Geometry check sheet. Reference: the model listing, model coordinates, mm. A direction names the side the tool comes from. Give positions to 0.01 mm unless a question says otherwise; leave off trailing zeros. Order: outer loops, then holes, each group sorted by start corner. A loop starts at its lowest first (then second) coordinate and runs counter-clockwise, first axis right, second up. Notation, with made-up numbers: M -10,63.25 L 35,63.25 A19 cw 35,86.25 Z; hole C 58.5,87 d5. An arc over 180 degrees is marked long. Answer as CSV lines item,"result". Start each with the question number.
Q1. Section check D-D, the plane x = 40. Record the boundary of the cut face in (y, z), then the cut area to 3 significant figures.
Q2. Mould release check, pull along Y, two halves, no side actions. Record for faces 4 (the cylindrical face through (4.4, 44.5, 1.2)), 5 (the flat face through (63, 2, 10)), 6 (the flat face through (20, 6.5, 10)): +Y half, -Y half, draft (parallel to the pull), parting line (faces both ways), or undercut.
Q3. Section check C-C, the plane z = 5.5. Record the boundary of the cut face in (x, y).
Q4. Section check B-B, the plane x = 4.5. Record the boundary of the cut face in (y, z).
Q5. Thickness scan on line 1 (Y direction, x = 4.5, z = 1.85); line 2 (X direction, y = 40, z = 19.25); line 3 (X direction, y = 7, z = 6.5). Record the ranges inside material, lowest first.
Q6. Set-up check for faces 1 (the flat face through (26, 25, 8)), 2 (the flat face through (18, 9, 10)), 3 (the flat face through (21, 9, 10)): record each of +Z, -Z, +X, -X, +Y, -Y from which the full face is reachable in a straight line by a thin tool's end or side.
Q7. Go/stop test with flat-tipped pins: pin 1 (4.5 mm diameter, centred on x = 19, z = 10.5, fed in from +Y); pin 2 (6.5 mm diameter, centred on x = 16.5, y = 9, fed in from +Z); pin 3 (3 mm diameter, centred on x = 61.5, z = 11, fed in from +Y); pin 4 (1 mm diameter, centred on x = 23, y = 25.5, fed in from +Z). Record where each tip stops, or that it passes through.
Q8. Section check A-A, the plane y = 22. Record the boundary of the cut face in (x, z).
Autodesk Inventor part; units mm, degrees
ref_plane "YZ Plane" through (0, 0, 0) normal (1, 0, 0) x (0, 1, 0)
ref_plane "XZ Plane" through (0, 0, 0) normal (0, 1, 0) x (-1, 0, 0)
ref_plane "XY Plane" through (0, 0, 0) normal (0, 0, 1) x (1, 0, 0)
sketch "Sketch1" plane through (0, 0, 0) normal (0, 0, 1) x (1, 0, 0)
  line L0 (0, 0) -> (0, 40)
  line L1 (0, 0) -> (63, 0)
  line L2 (63, 0) -> (63, 5)
  line L3 (63, 5) -> (9, 5)
  arc A0 (9, 40) -> (0, 40) centre (4.5, 40) ccw
  line L4 (9, 40) -> (9, 5)
  circle A1 centre (4.5, 40) radius 2.5
  dimension "d0" = 40
  dimension "d2" = 5
  dimension "d6" = 4.5
  dimension "d7" = 5
  dimension "d8" = 9
  dimension "d9" = 54
  dimension "d47" = 32.5
extrude "Extrusion1" add sketch "Sketch1" along normal blind 20
sketch "Sketch2" plane through (9, 5, 0) normal (0, 1, 0) x (1, 0, 0)
  line L0 (0, 0) -> (0, -20)
  circle A0 centre (26, -10) radius 10
  line L1 (0, 0) -> (54, 0)
  circle A1 centre (52, -10) radius 2
  line L2 (54, 0) -> (54, -20)
  point P0 (-9, 0)
  dimension "d14" = 20
  dimension "d16" = 26
  dimension "d20" = 4
  dimension "d21" = 10
  dimension "d22" = 14
sketch "Sketch6" plane through (9, 5, 0) normal (1, 0, 0) x (0, 0, -1)
  point P0 (0, -5)
sketch "Sketch7" plane through (9, 5, 0) normal (1, 0, 0) x (0, 0, -1)
  line L0 (-10, 41.0364) -> (-10, 39.6436)
  line L1 (0, 39.5) -> (-20, 39.5)
  line L2 (-2.5, 39.5) -> (-2.5, 25.5)
  line L3 (-17.5, 39.5) -> (-17.5, 25.5)
  line L4 (-17.5, 39.5) -> (-2.5, 39.5)
  line L5 (0, 32.5) -> (-20, 32.5)
  line L6 (-17.5, 25.5) -> (-2.5, 25.5)
  point P0 (0, -5)
  dimension "d40" = 14
  dimension "d41" = 14
  dimension "d42" = 15
extrude "Extrusion5" cut sketch "Sketch7" against normal blind 14
sketch "Sketch8" plane through (0, 0, 0) normal (0, 0, -1) x (-1, 0, 0)
  point P0 (0, 0)
extrude "Extrusion6" add sketch "Sketch2" along normal blind 20
sketch "Sketch9" plane through (35, 25, 10) normal (0, 1, 0) x (1, 0, 0)
  circle A0 centre (0, 0) radius 9
  point P0 (-35, 10)
  dimension "d50" = 18
extrude "Extrusion7" cut sketch "Sketch9" against normal blind 25
sketch "Sketch10" plane through (9, 5, 20) normal (0, 1, 0) x (1, 0, 0)
  line L0 (6, 8) -> (12, 8)
  line L1 (12, 8) -> (12, 12)
  line L2 (12, 12) -> (6, 12)
  line L3 (6, 12) -> (6, 8)
  line L4 (26, 0) -> (0, 0)
  line L5 (0, 2.5) -> (0, 17.5)
  point P0 (-9, 20)
  dimension "d53" = 6
  dimension "d54" = 4
  dimension "d55" = 8
  dimension "d56" = 6
extrude "Extrusion8" add sketch "Sketch10" along normal blind 6
sketch "Sketch11" plane through (21, 5, 8) normal (0, 0, -1) x (-1, 0, 0)
  line L0 (2, 4) -> (4, 4)
  line L1 (6, 0) -> (6, 6)
  line L2 (12, 0) -> (-14, 0)
  line L3 (0, 0) -> (6, 0)
  line L4 (0, 1.5) -> (0, 0)
  line L5 (6, 0) -> (0, 0)
  line L6 (0, 0) -> (3, 0)
  line L7 (0, 1.5) -> (2, 1.5)
  line L8 (2, 1.5) -> (2, 4)
  line L9 (3, 0) -> (0, 0)
  line L10 (4, 4) -> (4, 0)
  line L11 (0, 0) -> (6, 0)
  line L12 (0, 0) -> (4, 0)
  point P0 (21, -5)
  dimension "d59" = 2
  dimension "d60" = 2
  dimension "d61" = 4
  dimension "d62" = 1.5
extrude "Extrusion9" cut sketch "Sketch11" against normal blind 4
equation "\"d21\" = d19"
equation "\"d40\" = d41"
equation "\"d19\" = 0.5 * d14"
properties part number "ValveBaseMk2.3"
Answer block:
1,outline,"M 0,0 L 5,0 L 5,1.34 L 25,1.34 L 25,2.52 L 0,2.52 Z; M 0,17.48 L 25,17.48 L 25,18.66 L 5,18.66 L 5,20 L 0,20 Z"
1,area,"72.2 mm2"
2,face 4,"+Y half"
2,face 5,"draft"
2,face 6,"undercut"
3,outline,"M 0,0 L 27.21,0 L 27.21,25 L 26.07,25 L 26.07,5 L 9,5 L 9,30.5 L 0,30.5 Z; M 42.79,0 L 63,0 L 63,5 L 43.93,5 L 43.93,25 L 42.79,25 Z"
4,outline,"M 0,0 L 37.5,0 L 37.5,2.5 L 30.5,2.5 L 30.5,17.5 L 37.5,17.5 L 37.5,20 L 0,20 Z; M 42.5,0 L 44.5,0 L 44.5,2.5 L 42.5,2.5 Z; M 42.5,17.5 L 44.5,17.5 L 44.5,20 L 42.5,20 Z"
5,line 1,"y = 0 to 37.5, 42.5 to 44.5"
5,line 2,"x = 0 to 2, 7 to 9"
5,line 3,"x = 0 to 9, 25.63 to 26.71, 43.29 to 44.37"
6,face 1,"+Z, -Z, +X, +Y"
6,face 2,"+Z, -Z"
6,face 3,"+Z, -Z, +Y"
7,pin 1,"stops at y = 11"
7,pin 2,"stops at z = 12"
7,pin 3,"stops at y = 25"
7,pin 4,"passes through"
8,outline,"M 0,0 L 9,0 L 9,20 L 0,20 Z; C 35,10 d20; C 61,10 d4; hole C 35,10 d18"
